Could you check a few things on this drawing? It's one solid part, dimensions in mm from its lowest x, y, z. Give positions to 0.01 mm unless a question says otherwise; leave off trailing zeros. Order: outer loops, then holes, each group sorted by start corner. A loop starts at its lowest first (then second) coordinate and runs counter-clockwise, first axis right, second up. Notation, with made-up numbers: (28, -33) -> (86, -33) arc R35 cw to (86, 1) -> close; hole circle Ø3 at (-8.75, 75). An arc over 180 degrees is marked (long way). Write each question's results on one line, items separated by ' | '.
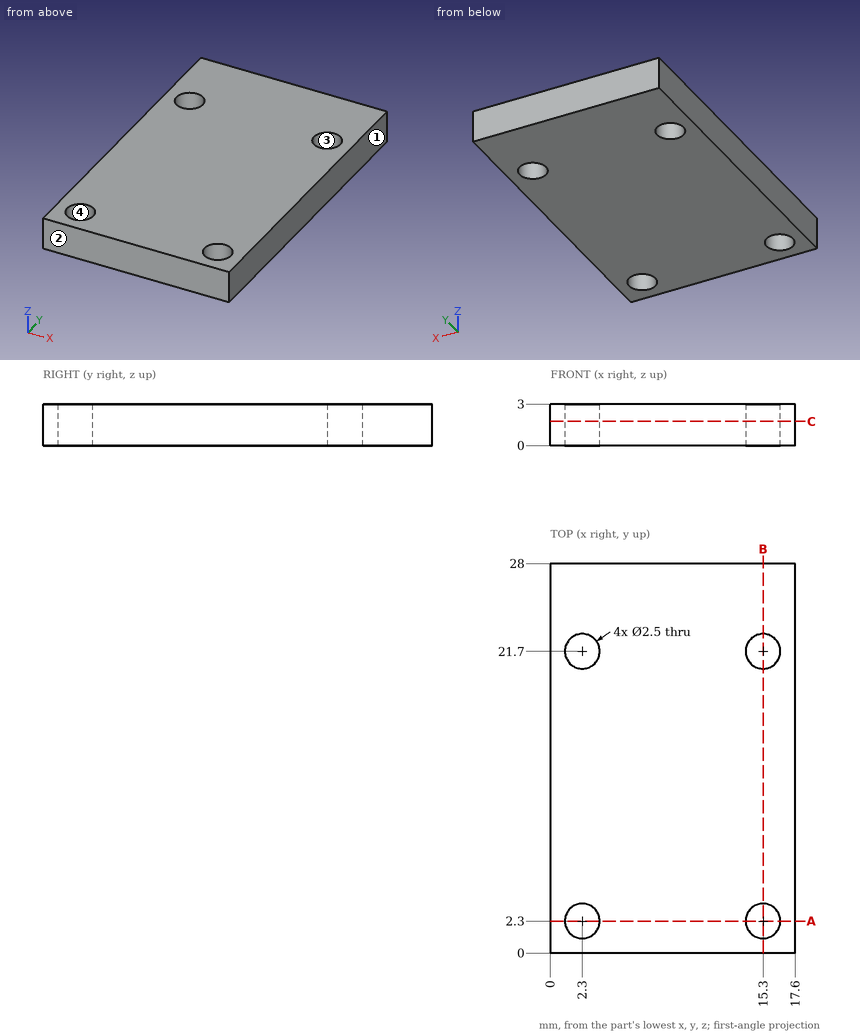
Q1. Suppose I cut it at A-A on y = 2.3. Please give me the cut outline in (x, z).
Here are the results:
outline: (0, 0) -> (1.05, 0) -> (1.05, 3) -> (0, 3) -> close; (3.55, 0) -> (14.05, 0) -> (14.05, 3) -> (3.55, 3) -> close; (16.55, 0) -> (17.6, 0) -> (17.6, 3) -> (16.55, 3) -> close
Q2. Suppose I cut it at B-B on x = 15.3. Please give me the cut outline in (y, z).
Here are the results:
outline: (0, 0) -> (1.05, 0) -> (1.05, 3) -> (0, 3) -> close; (3.55, 0) -> (20.45, 0) -> (20.45, 3) -> (3.55, 3) -> close; (22.95, 0) -> (28, 0) -> (28, 3) -> (22.95, 3) -> close
Q3. I need wall thicknesses on line 1 along Y through (x, z) = (15.3, 2.35); line 2 along Y through (x, z) = (14.5, 1.7); line 3 along X through (y, z) = (21.5, 0.9). Which ranges of each line are inside material? Lowest first, please.
Here are the results:
line 1: y = 0 to 1.05, 3.55 to 20.45, 22.95 to 28 | line 2: y = 0 to 1.34, 3.26 to 20.74, 22.66 to 28 | line 3: x = 0 to 1.07, 3.53 to 14.07, 16.53 to 17.6
Q4. Thinking about a two-plate mould opening in Y: for the marked faces 1, 2, 3 and 4, which applies, +Y half, -Y half, draft (parallel to the pull), parting line (faces both ways), or undercut?
Here are the results:
face 1: draft | face 2: -Y half | face 3: undercut | face 4: undercut
Q5. I'm going to push a flat-ended pin straight in: pin 1 Ø2 at (x, y) = (15.3, 21.7) entering from -Z. Where does the tip first touch, or does it pass through?
Here are the results:
pin 1: passes through
Q6. Suppose I cut it at C-C on z = 1.75. Please give me the cut outline in (x, y).
Here are the results:
outline: (0, 0) -> (17.6, 0) -> (17.6, 28) -> (0, 28) -> close; hole circle Ø2.5 at (2.3, 2.3); hole circle Ø2.5 at (2.3, 21.7); hole circle Ø2.5 at (15.3, 2.3); hole circle Ø2.5 at (15.3, 21.7)
